Can you work these out from the drawing? Everything is in mm from the part's minimum corner. Give positions to 0.01 mm unless a question says otherwise; leave off trailing zeros. Loops run counter-clockwise (first coordinate to the right, second up) from the corner with the lowest first, then second, coordinate; pieces in that order, holes last.
Q1. If we section it at C-C (z = 3.1): Give the number of separate pieces and of enclosed holes in the cut face.
Q2. I need wall thicknesses on line 1 (Y direction, x = 94.5, z = 1.1); line 2 (X direction, y = 90.5, z = 5.1); line 3 (X direction, y = 43, z = 5.65). Which ranges of each line are inside material? Lowest first, please.
Q3. If we section it at B-B (x = 23): Please give me the cut outline in (y, z), plus the area to 3 significant figures.
Q4. If we section it at A-A (y = 59): Please give me the cut outline in (x, z).
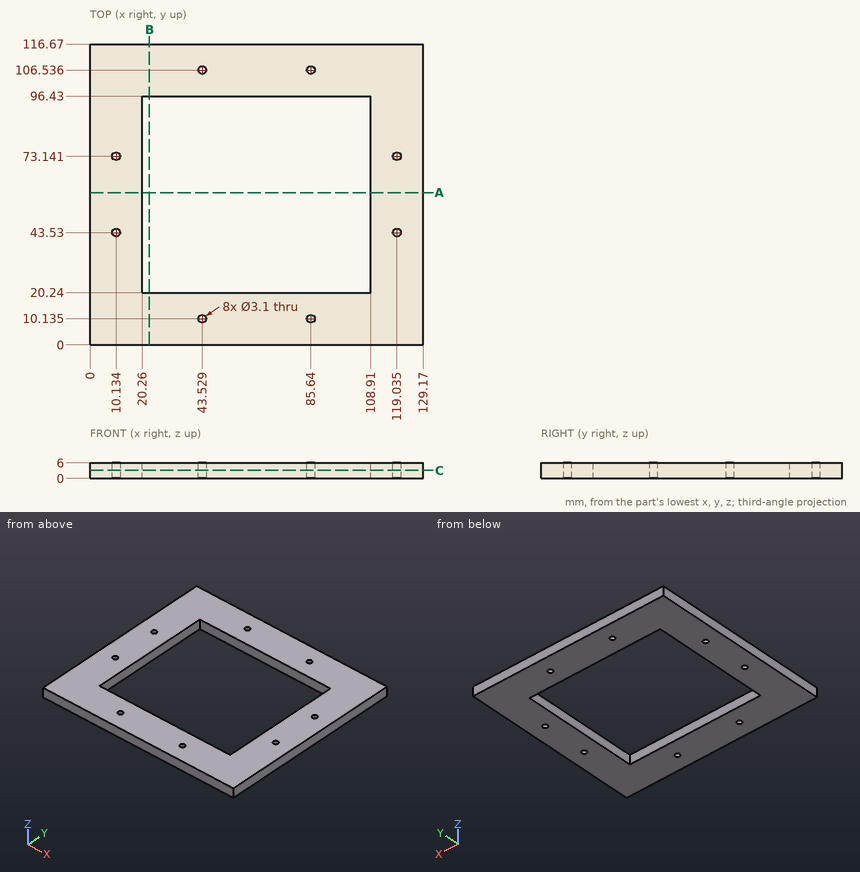
Check sheet entries:
1. separate pieces: 1
1. enclosed holes: 9
2. line 1: y = 0 to 20.24, 96.43 to 116.67
2. line 2: x = 0 to 20.26, 108.91 to 129.17
2. line 3: x = 0 to 8.68, 11.59 to 20.26, 108.91 to 117.58, 120.49 to 129.17
3. outline: (0, 0) - (20.24, 0) - (20.24, 6) - (0, 6) - close; (96.43, 0) - (116.67, 0) - (116.67, 6) - (96.43, 6) - close
3. area: 243 mm2
4. outline: (0, 0) - (20.26, 0) - (20.26, 6) - (0, 6) - close; (108.91, 0) - (129.17, 0) - (129.17, 6) - (108.91, 6) - close
